from build123d import *

# Parameters (mm, degrees)
SKETCH1_W           = 140
SKETCH1_H           = 140
BOSS_EXTRUDE1_DEPTH = 10
SKETCH2_R           = 5
BOSS_EXTRUDE2_DEPTH = 30


with BuildPart() as part:
    # Sketch1 → Boss-Extrude1 (new body)
    with BuildSketch(Plane.XY):
        Rectangle(SKETCH1_W, SKETCH1_H)
    extrude(amount=BOSS_EXTRUDE1_DEPTH)

    # Sketch2 → Boss-Extrude2 (add)
    with BuildSketch(Plane.XY):
        with Locations((-31.9, 0)):
            Circle(SKETCH2_R)
        with Locations((31.9, 0)):
            Circle(SKETCH2_R)
    extrude(amount=-BOSS_EXTRUDE2_DEPTH)


solid = part.part
Can you work these out from the model? Positions are in its coordinate system, mm. Coordinates: 2 decimals unless noted, no trailing zeros. Loops run counter-clockwise (first coordinate to the right, second up) from the corner with the lowest first, then second, coordinate; pieces in that order, holes last. Notation, with made-up numbers: M -13.5,-6.5 L 23.5,-6.5 A22 cw 23.5,6.5 Z; hole C 45,-12.75 d10. An arc over 180 degrees is marked long. Return JSON: item names as keys, results as strings. Group by question number.
Item 1: I'm going to push a flat-ended pin straight in: pin 1 Ø1.5 at (x, y) = (-21.5, -20) entering from -Z. Where does the tip first touch, or does it pass through?
Item 2: Imagine slicing it at D-D (x = 56.5). Please give me the cut outline in (y, z).
Item 3: Imagine slicing it at B-B (x = -31.9). Please give me the cut outline in (y, z).
Item 4: If I drill on L1, parallel to Z at x = -16.5, y = 34; L2, parallel to Y at x = -34, z = -25; L3, parallel to Y at x = -29.5, z = -24.5, over which ranges is the centre line in solid material (lowest first)? Write a range as from..to.
Item 5: Thinking about a two-plate mould opening in X: for faces 1 (the cylindrical face through (-36.895, 0.22, -14.79)), 2 (the cylindrical face through (26.905, 0.22, -14.79)), 3 (the flat face through (70, -1, 5)), 4 (the flat face through (-32, 0, -30)), which applies, released by +X, released by -X, zero draft, split by the parting line, or undercut?
Item 6: Imagine slicing it at C-C (z = -23.5). Please give me the cut outline in (x, y), and give its area (3 significant figures).
Item 7: Imagine slicing it at A-A (y = 0). Please give me the cut outline in (x, z).
Verdict:
{
 "1": {"pin 1": "stops at z = 0"},
 "2": {"outline": "M -70,0 L 70,0 L 70,10 L -70,10 Z"},
 "3": {"outline": "M -70,0 L -5,0 L -5,-30 L 5,-30 L 5,0 L 70,0 L 70,10 L -70,10 Z"},
 "4": {"L1": "z = 0..10", "L2": "y = -4.54..4.54", "L3": "y = -4.39..4.39"},
 "5": {"face 1": "undercut", "face 2": "undercut", "face 3": "released by +X", "face 4": "zero draft"},
 "6": {"outline": "C -31.9,0 d10; C 31.9,0 d10", "area": "157 mm^2"},
 "7": {"outline": "M -70,0 L -36.9,0 L -36.9,-30 L -26.9,-30 L -26.9,0 L 26.9,0 L 26.9,-30 L 36.9,-30 L 36.9,0 L 70,0 L 70,10 L -70,10 Z"}
}
